```python
from build123d import *

# Parameters (mm, degrees)
SKETCH003_R  = 4.75
PAD002_DEPTH = 8
PAD001_DEPTH = 4
SKETCH_R     = 6
PAD_DEPTH    = 4


with BuildPart() as trou:
    # Sketch003 → Pad002 (new body)
    with BuildSketch(Plane.XY):
        Circle(SKETCH003_R)
    extrude(amount=PAD002_DEPTH)


with BuildPart() as cylindre:
    # Sketch002 → Pad001 (new body)
    with BuildSketch(Plane.XY):
        Polygon((8.227241, 4.75), (0, 9.5), (-8.227241, 4.75), (-8.227241, -4.75), (0, -9.5), (8.227241, -4.75), align=None)
    extrude(amount=PAD001_DEPTH)


with BuildPart() as cut:
    # Sketch → Pad (new body)
    with BuildSketch(Plane.XY.offset(4)):
        Circle(SKETCH_R)
    extrude(amount=PAD_DEPTH)

    # Fusion: union cylindre
    add(cylindre.part)

    # Cut: cut trou
    add(trou.part, mode=Mode.SUBTRACT)


solid = cut.part
```
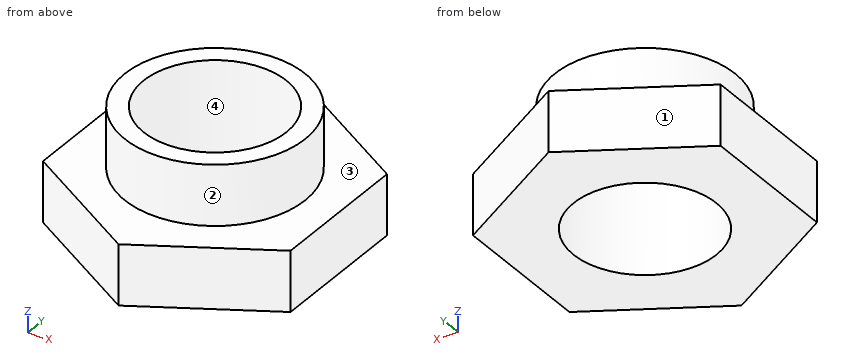
Can you work these out from the model? Positions are in its coordinate system, mm. Face numbers are marked on the shaded views. Give positions to 0.01 mm unless a question says otherwise; leave off trailing zeros. Order: outer loops, then holes, each group sorted by start corner. A loop starts at its lowest first (then second) coordinate and runs counter-clockwise, first axis right, second up. Notation, with made-up numbers: M -12.5,-24.75 L 22.5,-24.75 A29 cw 22.5,2.25 Z; hole C -6,27 d4. An arc over 180 degrees is marked long. Write item = value, one per line. Start each with the question number.
Q1. Suppose I cut it at A-A (y = 0). Write out the boundary of the cut face in (x, z), plus the area to 3 significant figures.
Q2. We'd pull the mould along X, two halves only. Please class the marked faces 1, 2, 3 and 4: pulls with the +X half, pulls with the -X half, needs draft (parallel to the pull), parting line crosses it, or undercut.
Q3. Will this pin go through, and if not, where does the flat tip stop? pin 1 Ø2 at (x, y) = (5, -6.5) entering from +Z.
Q4. Suppose I cut it at D-D (z = 6.5). Write out the boundary of the cut face in (x, y).
Q5. Suppose I cut it at B-B (z = 1.5). Write out the boundary of the cut face in (x, y), plus the area to 3 significant figures.
Q6. I need wall thicknesses on probe 1 along Y at (x, z) = (0, 4.5); probe 2 along X at (y, z) = (0.75, 6.25); probe 3 along X at (y, z) = (1, 1.5). Which ranges of each line are inside material? Lowest first, please. Write a range as [from, to].
Q7. Suppose I cut it at C-C (x = 1.75). Write out the boundary of the cut face in (y, z), plus the area to 3 significant figures.
Check result:
q1.outline = M -8.23,0 L -4.75,0 L -4.75,8 L -6,8 L -6,4 L -8.23,4 Z; M 4.75,0 L 8.23,0 L 8.23,4 L 6,4 L 6,8 L 4.75,8 Z
q1.area = 37.8 mm2
q2.face_1 = pulls with the -X half
q2.face_2 = parting line crosses it
q2.face_3 = needs draft
q2.face_4 = undercut
q3.pin_1 = 4
q4.outline = C 0,0 d12; hole C 0,0 d9.5
q5.outline = M -8.23,-4.75 L 0,-9.5 L 8.23,-4.75 L 8.23,4.75 L 0,9.5 L -8.23,4.75 Z; hole C 0,0 d9.5
q5.area = 164 mm2
q6.probe_1 = [-6, -4.75], [4.75, 6]
q6.probe_2 = [-5.95, -4.69], [4.69, 5.95]
q6.probe_3 = [-8.23, -4.64], [4.64, 8.23]
q7.outline = M -8.49,0 L -4.42,0 L -4.42,8 L -5.74,8 L -5.74,4 L -8.49,4 Z; M 4.42,0 L 8.49,0 L 8.49,4 L 5.74,4 L 5.74,8 L 4.42,8 Z
q7.area = 43.2 mm2
